```python
from build123d import *

# Parameters (mm, degrees)
BOSS_EXTRUDE1_DEPTH = 9.906
SKETCH3_R           = 6.35
BOSS_EXTRUDE2_DEPTH = 101.6
CHAMFER1_SIZE       = 0.9906


with BuildPart() as part:
    # Sketch1 → Boss-Extrude1 (new body)
    with BuildSketch(Plane(origin=(0, 0, 0), x_dir=(1, 0, 0), z_dir=(0, 1, 0))):
        Polygon((0, -11.73175747), (10.16, -5.865878735), (10.16, 5.865878735), (0, 11.73175747), (-10.16, 5.865878735), (-10.16, -5.865878735), align=None)
    extrude(amount=BOSS_EXTRUDE1_DEPTH)

    # Sketch3 → Boss-Extrude2 (add)
    with BuildSketch(Plane.XZ):
        with Locations(Location((0, 0, 0), (0, 0, 270))):
            Circle(SKETCH3_R)
    extrude(amount=BOSS_EXTRUDE2_DEPTH)

    # Chamfer1
    chamfer1_edges = [part.edges().sort_by_distance(p)[0] for p in [
        (0, -101.6, 6.35),
    ]]
    chamfer(chamfer1_edges, length=CHAMFER1_SIZE)

    # Sketch9 → Cut-Revolve4 (revolve, cut)
    with BuildSketch(Plane(origin=(0, 0, 0), x_dir=(0, 0, -1), z_dir=(1, 0, 0))):
        Polygon((-11.73175747, 9.906), (-10.46175747, 9.906), (-11.73175747, 8.89), align=None)
        Polygon((-11.73175747, 0), (-10.46175747, 0), (-11.73175747, 1.016), align=None)
    revolve(axis=Axis((0, 0, 0), (0, 1, 0)), mode=Mode.SUBTRACT)


solid = part.part
```
Source: CAD feature listing. Evaluate the final solid. Frame: model axes, mm. A direction names the side the tool comes from. Round coordinates to 2 decimals unless told otherwise and drop trailing zeros. Order: outer loops, then holes, each group sorted by start corner. A loop starts at its lowest first (then second) coordinate and runs counter-clockwise, first axis right, second up. Notation, with made-up numbers: (63, -18.5) -> (108, -18.5) arc R22 ccw to (108, -1.5) -> close; hole circle Ø11 at (-39.75, 20.25). An arc over 180 degrees is marked (long way). One line per item, written item: value. Start each with the question number.
Q1. Section query A-A (z = 0). Return the cut outline in (x, y).
Q2. Section query B-B (y = -19). Return the cut outline in (x, z), plus the area to 3 significant figures.
Q3. Material intervals for probe 1 along Z at (x, y) = (-0.5, -67.5); probe 2 along Y at (x, z) = (-6, 7.25), sorted ascending.
Q4. Access query for faces 1 (the cylindrical face through (-3.86, -49.6, 5.04)), 2 (the conical face through (-9.35, 9.62, -5.45)). Directions: +Z, -Z, +X, -X, +Y, -Y. A direction counts if a zero-diameter tool reaches every point of the face in a straight line with its end or side. Return the directions, or none.
Q5. Pin query (flat end, axial travel): pin 1 (6 mm diameter, centred on x = -0.5, y = -9.5, fed in from +Z); pin 2 (10 mm diameter, centred on x = 7.5, y = -43, fed in from +Z); pin 3 (12 mm diameter, centred on x = 5.5, z = -5.5, fed in from -Y); pin 4 (5 mm diameter, centred on x = 5.5, y = -6, fed in from +Z). Return the tip coordinate at first contact, or that it passes through.
Findings below:
1. outline: (-10.16, 0) -> (-6.35, 0) -> (-6.35, -100.61) -> (-5.36, -101.6) -> (5.36, -101.6) -> (6.35, -100.61) -> (6.35, 0) -> (10.16, 0) -> (10.16, 9.91) -> (-10.16, 9.91) -> close
2. outline: circle Ø12.7 at (0, 0)
2. area: 127 mm²
3. probe 1: -6.33 to 6.33
3. probe 2: 0 to 9.91
4. face 1: -Y
4. face 2: -Z, -X, +Y
5. pin 1: z = 6.35
5. pin 2: z = 5.84
5. pin 3: y = -101.6
5. pin 4: z = 5.6
